For this review, take the finished solid that the model builds, in its own axes (mm). A direction names the side the tool comes from. Round coordinates to 2 decimals unless told otherwise and drop trailing zeros. Order: outer loops, then holes, each group sorted by start corner. A loop starts at its lowest first (then second) coordinate and runs counter-clockwise, first axis right, second up. Notation, with made-up numbers: (50.25, 61.25) -> (77.25, 61.25) arc R14 cw to (77.25, 67.25) -> close; hole circle Ø9 at (-8, -37.5). An arc over 180 degrees is marked (long way). Use a Markdown table: item, result. Add a question column.
1) Consider section D-D (x = -35). State the section outline as (y, z) points (3 decimals).
2) Wall thickness on line 1 along X through (y, z) = (4.4, 6.39) (3 decimals); line 2 along Y through (x, z) = (7, 0) (3 decimals); line 3 along X through (y, z) = (-1, 2.25) (3 decimals): over which ranges is each line inside the solid? List them lowest first. Write a range as [from, to].
3) Draft analysis for pull direction Z (two halves, no side actions). For faces 1 (the face through (-40.195, 1, 0)), 2 (the face through (39.6, 4.03, 6.23)), 3 (the face through (-6.2, -6.4, 0.1)), 4 (the face through (38, 2, -6)), state which applies: pulls with the +Z half, pulls with the -Z half, needs draft (parallel to the pull), parting line crosses it, or undercut.
4) Clearance check with flat-ended pins moving along their axes: P1, Ø2, axis at x = 7, z = 1.5, coming from the -Y side; P2, Ø5, axis at y = -4.5, z = 0.5, coming from the +X side (3 decimals); P3, Ø2, axis at x = -20.5, z = 6, coming from the -Y side; P4, Ø6, axis at x = -20.5, y = -4.5, coming from the -Z side. State where each tip first meets the part, or that it passes through.
5) Machinability: for faces 5 (the face through (-7.715, -1.7, 0)), 6 (the face through (36.525, 1, 0)), 7 (the face through (7.715, -1.7, 0)), 8 (the face through (-1.543, -1.7, 0)), 9 (the face through (-39.469, 4.028, 6.967)), which of the approach directions +Z, -Z, +X, -X, +Y, -Y give a long, thin tool a straight path to every point of the face, cutting with its end or side? Answer none if there is none.
6) Consider section B-B (y = 0.75). State the section outline as (x, z) points (3 decimals), plus the area to 3 significant figures.
7) Consider section A-A (y = 3.75). State the section outline as (x, z) points (3 decimals), plus the area to 3 significant figures.
8) Consider section C-C (x = -12.5). State the section outline as (y, z) points (3 decimals), plus the area to 3 significant figures.
```python
from build123d import *

# Parameters (mm, degrees)
BOSS_EXTRUDE2_DEPTH = 2
SKETCH4_R           = 1.835
BOSS_EXTRUDE3_DEPTH = 4
SKETCH6_R           = 1.25
CUT_EXTRUDE1_DEPTH  = 4
SKETCH7_R           = 1.375
BOSS_EXTRUDE4_DEPTH = 3.086
LPATTERN1_COUNT     = 3
LPATTERN1_PITCH     = 6.172


with BuildPart() as part:
    # Sketch3 → Boss-Extrude2 (new body)
    with BuildSketch(Plane(origin=(0, 0, 0), x_dir=(1, 0, 0), z_dir=(0, 1, 0))):
        with BuildLine():
            Line((38.36, -8.225), (-38.36, -8.225))
            ThreePointArc((-38.36, -8.225), (-39.657541, -7.687541), (-40.195, -6.39))
            Line((-40.195, -6.39), (-40.195, 6.39))
            ThreePointArc((-40.195, 6.39), (-39.657541, 7.687541), (-38.36, 8.225))
            Line((-38.36, 8.225), (38.36, 8.225))
            ThreePointArc((38.36, 8.225), (39.657541, 7.687541), (40.195, 6.39))
            Line((40.195, 6.39), (40.195, -6.39))
            ThreePointArc((40.195, -6.39), (39.657541, -7.687541), (38.36, -8.225))
        make_face()
        Polygon((6.841855, -3), (27.192466, -6.39), (-27.192466, -6.39), (-6.841855, -3), align=None, mode=Mode.SUBTRACT)
        Polygon((-27.192466, 6.39), (-6.841855, 3), (6.841855, 3), (27.192466, 6.39), align=None, mode=Mode.SUBTRACT)
        Polygon((-36.525, 4.224041), (-36.525, -4.224041), (-11.167534, 0), align=None, mode=Mode.SUBTRACT)
        Polygon((36.525, -4.224041), (11.167534, 0), (36.525, 4.224041), align=None, mode=Mode.SUBTRACT)
    extrude(amount=BOSS_EXTRUDE2_DEPTH)

    # Sketch4 → Boss-Extrude3 (add)
    with BuildSketch(Plane(origin=(0, 2, 0), x_dir=(1, 0, 0), z_dir=(0, 1, 0))):
        with Locations(Location((-38.36, 6.39, 0), (0, 0, 90))):
            Circle(SKETCH4_R)
        with Locations(Location((-38.36, -6.39, 0), (0, 0, 270))):
            Circle(SKETCH4_R)
        with Locations(Location((38.36, 6.39, 0), (0, 0, 90))):
            Circle(SKETCH4_R)
        with Locations(Location((38.36, -6.39, 0), (0, 0, 270))):
            Circle(SKETCH4_R)
    extrude(amount=BOSS_EXTRUDE3_DEPTH)

    # Sketch6 → Cut-Extrude1 (cut)
    with BuildSketch(Plane(origin=(0, 6, 0), x_dir=(1, 0, 0), z_dir=(0, 1, 0))):
        with Locations(Location((-38.36, 6.39, 0), (0, 0, 270))):
            Circle(SKETCH6_R)
        with Locations(Location((-38.36, -6.39, 0), (0, 0, 270))):
            Circle(SKETCH6_R)
        with Locations(Location((38.36, 6.39, 0), (0, 0, 270))):
            Circle(SKETCH6_R)
        with Locations(Location((38.36, -6.39, 0), (0, 0, 270))):
            Circle(SKETCH6_R)
    extrude(amount=-CUT_EXTRUDE1_DEPTH, mode=Mode.SUBTRACT)

    # Sketch7 → Boss-Extrude4 (add)
    with BuildSketch(Plane.ZY.offset(-7.715)):
        with BuildLine():
            Line((-3, 0), (3, 0))
            Line((3, 0), (3, -3.4))
            ThreePointArc((3, -3.4), (0, -6.4), (-3, -3.4))
            Line((-3, -3.4), (-3, 0))
        make_face()
        with Locations((0, -3.4)):
            Circle(SKETCH7_R, mode=Mode.SUBTRACT)
    boss_extrude4 = extrude(amount=BOSS_EXTRUDE4_DEPTH)

    # LPattern1: Boss-Extrude4 ×3
    with Locations(*[(-i * LPATTERN1_PITCH, 0, 0) for i in range(1, LPATTERN1_COUNT)]):
        add(boss_extrude4)


solid = part.part
```
Results list:
| question | item | result |
|---|---|---|
| 1 | outline | (0, -8.225) -> (2, -8.225) -> (2, -3.97) -> (0, -3.97) -> close; (0, 3.97) -> (2, 3.97) -> (2, 8.225) -> (0, 8.225) -> close |
| 2 | line 1 | [-40.195, -39.61], [-37.11, -36.525], [36.525, 37.11], [39.61, 40.195] |
| 2 | line 2 | [-6.4, -4.775], [-2.025, 2] |
| 2 | line 3 | [-7.715, -4.629], [-1.543, 1.543], [4.629, 7.715] |
| 3 | face 1 | needs draft |
| 3 | face 2 | undercut |
| 3 | face 3 | parting line crosses it |
| 3 | face 4 | undercut |
| 4 | P1 | y = -6.36 |
| 4 | P2 | x = 7.715 |
| 4 | P3 | y = 0 |
| 4 | P4 | through |
| 5 | face 5 | +Z, -Z, -X, -Y |
| 5 | face 6 | +Y, -Y |
| 5 | face 7 | +Z, -Z, +X, -Y |
| 5 | face 8 | +Z, -Z, -Y |
| 5 | face 9 | +Y |
| 6 | outline | (-40.195, -6.39) arc R1.835 ccw to (-38.36, -8.225) -> (38.36, -8.225) arc R1.835 ccw to (40.195, -6.39) -> (40.195, 6.39) arc R1.835 ccw to (38.36, 8.225) -> (-38.36, 8.225) arc R1.835 ccw to (-40.195, 6.39) -> close; hole (-36.525, -4.224) -> (-11.168, 0) -> (-36.525, 4.224) -> close; hole (-27.192, -6.39) -> (27.192, -6.39) -> (6.842, -3) -> (-6.842, -3) -> close; hole (-27.192, 6.39) -> (-6.842, 3) -> (6.842, 3) -> (27.192, 6.39) -> close; hole (11.168, 0) -> (36.525, -4.224) -> (36.525, 4.224) -> close |
| 6 | area | 875 mm2 |
| 7 | outline | circle Ø3.67 at (-38.36, -6.39); circle Ø3.67 at (-38.36, 6.39); circle Ø3.67 at (38.36, -6.39); circle Ø3.67 at (38.36, 6.39); hole circle Ø2.5 at (-38.36, -6.39); hole circle Ø2.5 at (-38.36, 6.39); hole circle Ø2.5 at (38.36, -6.39); hole circle Ø2.5 at (38.36, 6.39) |
| 7 | area | 22.7 mm2 |
| 8 | outline | (0, -8.225) -> (2, -8.225) -> (2, -6.39) -> (0, -6.39) -> close; (0, -3.943) -> (2, -3.943) -> (2, -0.222) -> (0, -0.222) -> close; (0, 0.222) -> (2, 0.222) -> (2, 3.943) -> (0, 3.943) -> close; (0, 6.39) -> (2, 6.39) -> (2, 8.225) -> (0, 8.225) -> close |
| 8 | area | 22.2 mm2 |
